from build123d import *

# Parameters (mm, degrees)
F0_R     = 5
F1_DEPTH = 3


with BuildPart() as f1:
    # F0 (on Top) → F1 (new body)
    with BuildSketch(Plane.XY):
        with BuildLine():
            Line((-105.220296, 49.665504), (-140.720296, 49.665504))
            ThreePointArc((-140.720296, 49.665504), (-142.13451, 49.079717), (-142.720296, 47.665504))
            Line((-142.720296, 47.665504), (-142.720296, -27.334496))
            ThreePointArc((-142.720296, -27.334496), (-142.13451, -28.74871), (-140.720296, -29.334496))
            Line((-140.720296, -29.334496), (-122.720296, -29.334496))
            Line((-122.720296, -29.334496), (-122.720296, -95.334496))
            ThreePointArc((-122.720296, -95.334496), (-122.13451, -96.74871), (-120.720296, -97.334496))
            Line((-120.720296, -97.334496), (-35.720296, -97.334496))
            ThreePointArc((-35.720296, -97.334496), (-34.306083, -96.74871), (-33.720296, -95.334496))
            Line((-33.720296, -95.334496), (-33.720296, -29.334496))
            Line((-33.720296, -29.334496), (-15.720296, -29.334496))
            ThreePointArc((-15.720296, -29.334496), (-14.306083, -28.74871), (-13.720296, -27.334496))
            Line((-13.720296, -27.334496), (-13.720296, 47.665504))
            ThreePointArc((-13.720296, 47.665504), (-14.306083, 49.079717), (-15.720296, 49.665504))
            Line((-15.720296, 49.665504), (-51.220296, 49.665504))
            ThreePointArc((-51.220296, 49.665504), (-52.63451, 49.079717), (-53.220296, 47.665504))
            Line((-53.220296, 47.665504), (-53.220296, 15.665504))
            ThreePointArc((-53.220296, 15.665504), (-78.220296, -9.334496), (-103.220296, 15.665504))
            Line((-103.220296, 15.665504), (-103.220296, 47.665504))
            ThreePointArc((-103.220296, 47.665504), (-103.806083, 49.079717), (-105.220296, 49.665504))
        make_face()
        with Locations((-110.220296, -87.334496)):
            Circle(F0_R, mode=Mode.SUBTRACT)
        with Locations((-46.220296, -87.334496)):
            Circle(F0_R, mode=Mode.SUBTRACT)
        Polygon((-120.220296, 37.565504), (-118.220296, 37.565504), (-118.220296, 35.565504), (-118.220296, -10.434496), (-118.220296, -12.434496), (-120.220296, -12.434496), (-125.220296, -12.434496), (-127.220296, -12.434496), (-127.220296, -10.434496), (-127.220296, 35.565504), (-127.220296, 37.565504), (-125.220296, 37.565504), align=None, mode=Mode.SUBTRACT)
        with BuildLine():
            ThreePointArc((-38.220296, 35.565504), (-37.63451, 36.979717), (-36.220296, 37.565504))
            Line((-36.220296, 37.565504), (-31.220296, 37.565504))
            ThreePointArc((-31.220296, 37.565504), (-29.806083, 36.979717), (-29.220296, 35.565504))
            Line((-29.220296, 35.565504), (-29.220296, -10.434496))
            ThreePointArc((-29.220296, -10.434496), (-29.806083, -11.84871), (-31.220296, -12.434496))
            Line((-31.220296, -12.434496), (-36.220296, -12.434496))
            ThreePointArc((-36.220296, -12.434496), (-37.63451, -11.84871), (-38.220296, -10.434496))
            Line((-38.220296, -10.434496), (-38.220296, 35.565504))
        make_face(mode=Mode.SUBTRACT)
    extrude(amount=F1_DEPTH)


solid = f1.part
Check sheet for the modelled part. Datum: model origin and axes. Units: mm. A direction names the side the tool comes from. Give positions to 0.01 mm unless a question says otherwise; leave off trailing zeros. Write each loop counter-clockwise with the first axis right and the second up, starting at its lowest first coordinate (ties: lowest second). Pieces come first, ordered by that corner, then holes. Notation, with made-up numbers: M -33.5,49.25 L 16.5,49.25 A20 ccw 16.5,64.25 Z; hole C -18,58 d3. An arc over 180 degrees is marked long. Use one line per item in the form item = value.
(1) Section check B-B on x = -107. Record the boundary of the cut face in (y, z).
Answer block:
outline = M -97.33,0 L -91.16,0 L -91.16,3 L -97.33,3 Z; M -83.51,0 L 49.67,0 L 49.67,3 L -83.51,3 Z
(2) Section check A-A on y = 18. Record the boundary of the cut face in (x, z).
Answer block:
outline = M -142.72,0 L -127.22,0 L -127.22,3 L -142.72,3 Z; M -118.22,0 L -103.22,0 L -103.22,3 L -118.22,3 Z; M -53.22,0 L -38.22,0 L -38.22,3 L -53.22,3 Z; M -29.22,0 L -13.72,0 L -13.72,3 L -29.22,3 Z
(3) Tool access check on faces 5 (the flat face through (-25, -29.334, 1)), 6 (the flat face through (-29.22, 13, 1)), 7 (the flat face through (-132, -29.334, 1)), 8 (the flat face through (-103.22, 31, 1)). Record the directions out of +Z, -Z, +X, -X, +Y, -Y that give a thin tool (end or side, any length) a straight path to the whole face; none if there is none.
Answer block:
face_5 = +Z, -Z, +X, -Y
face_6 = +Z, -Z
face_7 = +Z, -Z, -X, -Y
face_8 = +Z, -Z, +Y
(4) Section check C-C on z = 0.7. State how many separate pieces and enclosed holes the cut face has, plus the area to 3 significant figures.
Answer block:
separate_pieces = 1
enclosed_holes = 4
area = 12,500 mm2
(5) Section check D-D on x = -129. Record the boundary of the cut face in (y, z), plus the area to 3 significant figures.
Answer block:
outline = M -29.33,0 L 49.67,0 L 49.67,3 L -29.33,3 Z
area = 237 mm2
(6) Material ranges on line 1 along X through (y, z) = (34.5, 1.7); line 2 along X through (y, z) = (42, 1.1); line 3 along X through (y, z) = (-85, 1.75), recorded low to high.
Answer block:
line_1 = -142.72 to -127.22, -118.22 to -103.22, -53.22 to -38.22, -29.22 to -13.72
line_2 = -142.72 to -103.22, -53.22 to -13.72
line_3 = -122.72 to -114.64, -105.8 to -50.64, -41.8 to -33.72
(7) Draft check along X on faces 1 (the flat face through (-142.72, 11, 1)), 2 (the flat face through (-53.22, 32, 1)), 3 (the flat face through (-79, -23, 0)), 4 (the flat face through (-13.72, 10, 1)). Enter one of: pulls with the +X half, pulls with the -X half, needs draft (parallel to the pull), parting line crosses it, or undercut.
Answer block:
face_1 = pulls with the -X half
face_2 = undercut
face_3 = needs draft
face_4 = pulls with the +X half
(8) Depth check by flat-ended pin: P1, Ø12, axis at x = -88.5, y = -9.5, coming from the -Z side; P2, Ø0.9, axis at x = -124.5, z = 1.5, coming from the -Y side; P3, Ø1.5, axis at y = -72.5, z = 2, coming from the +X side. Enter the tip coordinate at first touch or a pass-through.
Answer block:
P1 = 0
P2 = -29.33
P3 = -33.72
